from build123d import *

# Parameters (mm, degrees)
SKETCH1_W              = 30
SKETCH1_H              = 20
BOSS_EXTRUDE1_DEPTH    = 6
M3_CLEARANCE_HOLE1_D   = 3.2
SKETCH234_W            = 10
SKETCH234_H            = 6
BOSS_EXTRUDE234_DEPTH  = 6
FILLET134_R            = 1
SKETCH2342_W           = 10
SKETCH2342_H           = 6
BOSS_EXTRUDE2342_DEPTH = 6
FILLET1342_R           = 1


with BuildPart() as part:
    # Sketch1 → Boss-Extrude1 (new body)
    with BuildSketch(Plane(origin=(0, 0, 0), x_dir=(1, 0, 0), z_dir=(0, 1, 0))):
        Rectangle(SKETCH1_W, SKETCH1_H)
    extrude(amount=BOSS_EXTRUDE1_DEPTH)

    # M3 Clearance Hole1 (through all)
    with Locations(Plane(origin=(0, 6, 0), x_dir=(1, 0, 0), z_dir=(0, 1, 0))):
        with Locations((-9.275, 0), (9.775, 0)):
            Hole(M3_CLEARANCE_HOLE1_D / 2)

    # Sketch234 → Boss-Extrude234 (add)
    with BuildSketch(Plane(origin=(-15, 6, 0.767778608), x_dir=(0, 0, -1), z_dir=(-1, 0, 0))):
        with Locations((0.767778608, 3)):
            Rectangle(SKETCH234_W, SKETCH234_H)
    extrude(amount=BOSS_EXTRUDE234_DEPTH)

    # Fillet134
    fillet134_edges = [part.edges().sort_by_distance(p)[0] for p in [
        (-21, 3, 5),
        (-21, 3, -5),
    ]]
    fillet(fillet134_edges, radius=FILLET134_R)

    # Sketch2342 → Boss-Extrude2342 (add)
    with BuildSketch(Plane(origin=(-0.767778608, 6, -10), x_dir=(1, 0, 0), z_dir=(0, 0, -1))):
        with Locations((0.767778608, 3)):
            Rectangle(SKETCH2342_W, SKETCH2342_H)
    extrude(amount=BOSS_EXTRUDE2342_DEPTH)

    # Fillet1342
    fillet1342_edges = [part.edges().sort_by_distance(p)[0] for p in [
        (-5, 3, -16),
        (5, 3, -16),
    ]]
    fillet(fillet1342_edges, radius=FILLET1342_R)


solid = part.part
Geometry: final body of the model. Coordinates: model frame, mm. A direction names the side the tool comes from. Give positions to 0.01 mm unless a question says otherwise; leave off trailing zeros. Loops run counter-clockwise (first coordinate to the right, second up) from the corner with the lowest first, then second, coordinate; pieces in that order, holes last. Notation, with made-up numbers: M 39,-3 L 93,-3 A38 ccw 93,35 Z; hole C 13,39.25 d3. An arc over 180 degrees is marked long. Put each result on its own line as item: value. Start each with the question number.
1) Access query for faces 1 (the flat face through (-17, 3, -5)), 2 (the flat face through (-15, 3, 8)), 3 (the flat face through (10, 3, -10)). Directions: +Z, -Z, +X, -X, +Y, -Y. A direction counts if a zero-diameter tool reaches every point of the face in a straight line with its end or side. Return the directions, or none.
2) Pull-direction query (Z, two-part tool) for faces 4 (the flat face through (15, 3, 0)), 5 (the flat face through (0, 3, -16)), 6 (the cylindrical face through (-8.005, 2.958, 0.974)), 7 (the cylindrical face through (11.373, 2.958, -0.07)); classes: pulls with the +Z half, pulls with the -Z half, needs draft (parallel to the pull), parting line crosses it, or undercut.
3) Cut plane D-D (z = 7.25). Output: boundary loops of the cut face in (x, y), then the cut area to 3 significant figures.
4) Ray query, line 1 along X through (y, z) = (1.4, -9); line 2 along Z through (x, y) = (-11, 4.65); line 3 along Z through (x, y) = (9.5, 5.5). Return the intervals inside material, ascending.
5) Cut plane C-C (x = -14.5). Output: boundary loops of the cut face in (y, z), then the cut area to 3 significant figures.
6) Cut plane A-A (z = 0). Output: boundary loops of the cut face in (x, y) (3 decimals).
7) Contact query for flat-ended pins moving along their axis: pin 1 (1 mm diameter, centred on x = -17, y = 5.5, fed in from -Z); pin 2 (1.5 mm diameter, centred on y = 4, z = -11.5, fed in from +X). Output: stop coordinate, or through.
8) Cut plane B-B (y = 4.3). Output: boundary loops of the cut face in (x, z) (3 decimals), then the cut area to 3 significant figures.
Verdict:
1. face 1: -Z, -X, +Y, -Y
1. face 2: +Z, -X, +Y, -Y
1. face 3: -Z, +X, +Y, -Y
2. face 4: needs draft
2. face 5: pulls with the -Z half
2. face 6: undercut
2. face 7: undercut
3. outline: M -15,0 L 15,0 L 15,6 L -15,6 Z
3. area: 180 mm2
4. line 1: -15 to 15
4. line 2: -10 to 10
4. line 3: -10 to -1.58, 1.58 to 10
5. outline: M 0,-10 L 6,-10 L 6,10 L 0,10 Z
5. area: 120 mm2
6. outline: M -21,0 L -10.875,0 L -10.875,6 L -21,6 Z; M -7.675,0 L 8.175,0 L 8.175,6 L -7.675,6 Z; M 11.375,0 L 15,0 L 15,6 L 11.375,6 Z
7. pin 1: z = -5
7. pin 2: x = 5
8. outline: M -21,-4 A1 ccw -20,-5 L -15,-5 L -15,-10 L -5,-10 L -5,-15 A1 ccw -4,-16 L 4,-16 A1 ccw 5,-15 L 5,-10 L 15,-10 L 15,10 L -15,10 L -15,5 L -20,5 A1 ccw -21,4 Z; hole C -9.275,0 d3.2; hole C 9.775,0 d3.2
8. area: 703 mm2
